Work out the finished part from the listing and answer in its coordinate system (mm). A direction names the side the tool comes from. Coordinates: 2 decimals unless noted, no trailing zeros. Order: outer loops, then holes, each group sorted by start corner. A loop starts at its lowest first (then second) coordinate and runs counter-clockwise, first axis right, second up. Notation, with made-up numbers: M 22.5,71.5 L 69.5,71.5 A33 ccw 69.5,109.5 Z; hole C 60,70.5 d7. An arc over 180 degrees is marked long. Use a Markdown table: item, result.
from build123d import *

# Parameters (mm, degrees)
SKETCH1_R           = 2.1
BOSS_EXTRUDE1_DEPTH = 6
SKETCH2_R           = 2.1
BOSS_EXTRUDE2_DEPTH = 9
SKETCH3_W           = 5
SKETCH3_H           = 58.48
CUT_EXTRUDE1_DEPTH  = 16


with BuildPart() as part:
    # Sketch1 → Boss-Extrude1 (new body)
    with BuildSketch(Plane(origin=(0, 0, 0), x_dir=(1, 0, 0), z_dir=(0, 1, 0))):
        with BuildLine():
            Line((22.603957871, 7.564350825), (1.952968403, 14.673263119))
            ThreePointArc((1.952968403, 14.673263119), (0.990055879, 14.917752053), (0, 15))
            Line((0, 15), (0, -15))
            ThreePointArc((0, -15), (2.077420969, -14.818812213), (4.092108053, -14.280720353))
            Line((4.092108053, -14.280720353), (22.728072035, -7.520480235))
            ThreePointArc((22.728072035, -7.520480235), (27.999729231, 0.065819743), (22.603957871, 7.564350825))
        make_face()
        with Locations((20, 0)):
            Circle(SKETCH1_R, mode=Mode.SUBTRACT)
    boss_extrude1 = extrude(amount=BOSS_EXTRUDE1_DEPTH)

    # Mirror1: Boss-Extrude1 across plane
    add(boss_extrude1.mirror(Plane(origin=(0, 6, -15), x_dir=(0, 0, 1), z_dir=(1, 0, 0))))

    # Sketch2 → Boss-Extrude2 (add, symmetric)
    with BuildSketch(Plane(origin=(0, 0, 0), x_dir=(0, 0, -1), z_dir=(1, 0, 0))):
        with BuildLine():
            Line((-10, 6), (-3.895258642, 32.149373472))
            ThreePointArc((-3.895258642, 32.149373472), (0, 35.24), (3.895258642, 32.149373472))
            Line((3.895258642, 32.149373472), (10, 6))
            Line((10, 6), (-10, 6))
        make_face()
        with Locations((0, 31.24)):
            Circle(SKETCH2_R, mode=Mode.SUBTRACT)
    extrude(amount=BOSS_EXTRUDE2_DEPTH, both=True)

    # Sketch3 → Cut-Extrude1 (cut, symmetric)
    with BuildSketch(Plane.XY):
        with Locations((-5, 35.24)):
            Rectangle(SKETCH3_W, SKETCH3_H)
    cut_extrude1 = extrude(amount=CUT_EXTRUDE1_DEPTH, both=True, mode=Mode.SUBTRACT)

    # Mirror2: Cut-Extrude1 across plane
    add(cut_extrude1.mirror(Plane(origin=(0, 0, 0), x_dir=(0, 0, 1), z_dir=(1, 0, 0))), mode=Mode.SUBTRACT)


solid = part.part
(1) Determine the mould class of faces 6 (the cylindrical face through (8.26, 35.24, 0.08)), 7 (the cylindrical face through (-8.3, 29.2, 0.5)), 8 (the cylindrical face through (28, 3, 0)) for opening direction Y: pulls with the +Y half, pulls with the -Y half, needs draft (parallel to the pull), parting line crosses it, or undercut.
Conclusion:
| item | result |
|---|---|
| face 6 | pulls with the +Y half |
| face 7 | undercut |
| face 8 | needs draft |
(2) A cutting plane is placed at C-C (y = 31.24). Determine the outline of the cut face in (x, z).
Conclusion:
| item | result |
|---|---|
| outline | M -9,-4.11 L -7.5,-4.11 L -7.5,-2.1 L -9,-2.1 Z; M -9,2.1 L -7.5,2.1 L -7.5,4.11 L -9,4.11 Z; M -2.5,-4.11 L 2.5,-4.11 L 2.5,-2.1 L -2.5,-2.1 Z; M -2.5,2.1 L 2.5,2.1 L 2.5,4.11 L -2.5,4.11 Z; M 7.5,-4.11 L 9,-4.11 L 9,-2.1 L 7.5,-2.1 Z; M 7.5,2.1 L 9,2.1 L 9,4.11 L 7.5,4.11 Z |
(3) A cutting plane is placed at B-B (y = 11). Determine the outline of the cut face in (x, z).
Conclusion:
| item | result |
|---|---|
| outline | M -9,-8.83 L -7.5,-8.83 L -7.5,8.83 L -9,8.83 Z; M -2.5,-8.83 L 2.5,-8.83 L 2.5,8.83 L -2.5,8.83 Z; M 7.5,-8.83 L 9,-8.83 L 9,8.83 L 7.5,8.83 Z |
(4) A cutting plane is placed at D-D (z = 0). Give the number of separate pieces and of enclosed holes in the cut face, then the cut area to 3 significant figures.
Conclusion:
| item | result |
|---|---|
| separate pieces | 6 |
| enclosed holes | 0 |
| area | 486 mm2 |
(5) Which of the six approach directions +Z, -Z, +X, -X, +Y, -Y give full straight-line access (tool end or side, diameter ignored) to faces 1 (the flat face through (8.26, 19.258, -6.905)), 2 (the flat face through (2.5, 17, 0)), 3 (the flat face through (9, 18, 0)), 4 (the flat face through (-9, 18, 0)), 5 (the flat face through (0, 0, 0))?
Conclusion:
| item | result |
|---|---|
| face 1 | -Z, +X, -X, +Y |
| face 2 | +Z, -Z, +Y |
| face 3 | +Z, -Z, +X, +Y |
| face 4 | +Z, -Z, -X, +Y |
| face 5 | +Z, -Z, +X, -X, -Y |
(6) Given P1, Ø5, axis at x = 7, y = 7, coming from the +Z side; P2, Ø10, axis at y = 26, z = 4, coming from the +X side; P3, Ø9, axis at x = 7, z = 5, coming from the +Y side (3 decimals); P4, Ø2, axis at x = -4, y = 20.5, coming from the +Z side, each flat-ended and moving along its own axis, determine where each tip first touches the part or whether it passes through.
Conclusion:
| item | result |
|---|---|
| P1 | z = 14.06 |
| P2 | x = 9 |
| P3 | y = 35.205 |
| P4 | through |
(7) A cutting plane is placed at A-A (x = -20). Determine the outline of the cut face in (y, z), then the cut area to 3 significant figures.
Conclusion:
| item | result |
|---|---|
| outline | M 0,-8.46 L 6,-8.46 L 6,-2.1 L 0,-2.1 Z; M 0,2.1 L 6,2.1 L 6,8.51 L 0,8.51 Z |
| area | 76.6 mm2 |
(8) Straight lines are drawn through the part: L1, parallel to X at y = 15.5, z = -0.5; L2, parallel to X at y = 1.8, z = 0; L3, parallel to Y at x = -8, z = 0. For each, find the intervals that lie inside material, in ascending order.
Conclusion:
| item | result |
|---|---|
| L1 | -9 to -7.5, -2.5 to 2.5, 7.5 to 9 |
| L2 | -28 to -22.1, -17.9 to 17.9, 22.1 to 28 |
| L3 | 0 to 29.14, 33.34 to 35.24 |
